Answer from the drawing. Dimensions are ordinates in mm from the lowest x, y and z of the part. A direction names the side the tool comes from. Give positions to 0.01 mm unless a question says otherwise; leave off trailing zeros. Loops run counter-clockwise (first coordinate to the right, second up) from the corner with the lowest first, then second, coordinate; pieces in that order, holes last.
(1) Find section B-B, the plane x = 7.5. Write down the section's boundary in (y, z), then the cut area to 3 significant figures.
(2) Each of these flat-tipped pins is pushed along its axis until it touches: P1, Ø2, axis at x = 8, z = 9, coming from the +Y side; P2, Ø5, axis at x = 7.5, z = 9.5, coming from the +Y side; P3, Ø1, axis at y = 7.5, z = 3, coming from the -X side; P4, Ø1.5, axis at x = 9.5, y = 4, coming from the -Z side. Where does it stop, or does it pass through?
(3) Find section C-C, the plane z = 10. Write down the section's boundary in (x, y).
(4) Which of the six approach directions +Z, -Z, +X, -X, +Y, -Y give full straight-line access (tool end or side, diameter ignored) to the marked faces 1 and 2?
(5) Straight lines are drawn through the part: probe 1 along Z at (x, y) = (10.5, 4); probe 2 along Y at (x, z) = (9.25, 3); probe 3 along X at (y, z) = (2.75, 3.5). For each, find the intervals that lie inside material, in ascending order.
(6) Find section D-D, the plane y = 8.5. Write down the section's boundary in (x, z).
(7) Find section A-A, the plane y = 6.5. Write down the section's boundary in (x, z).
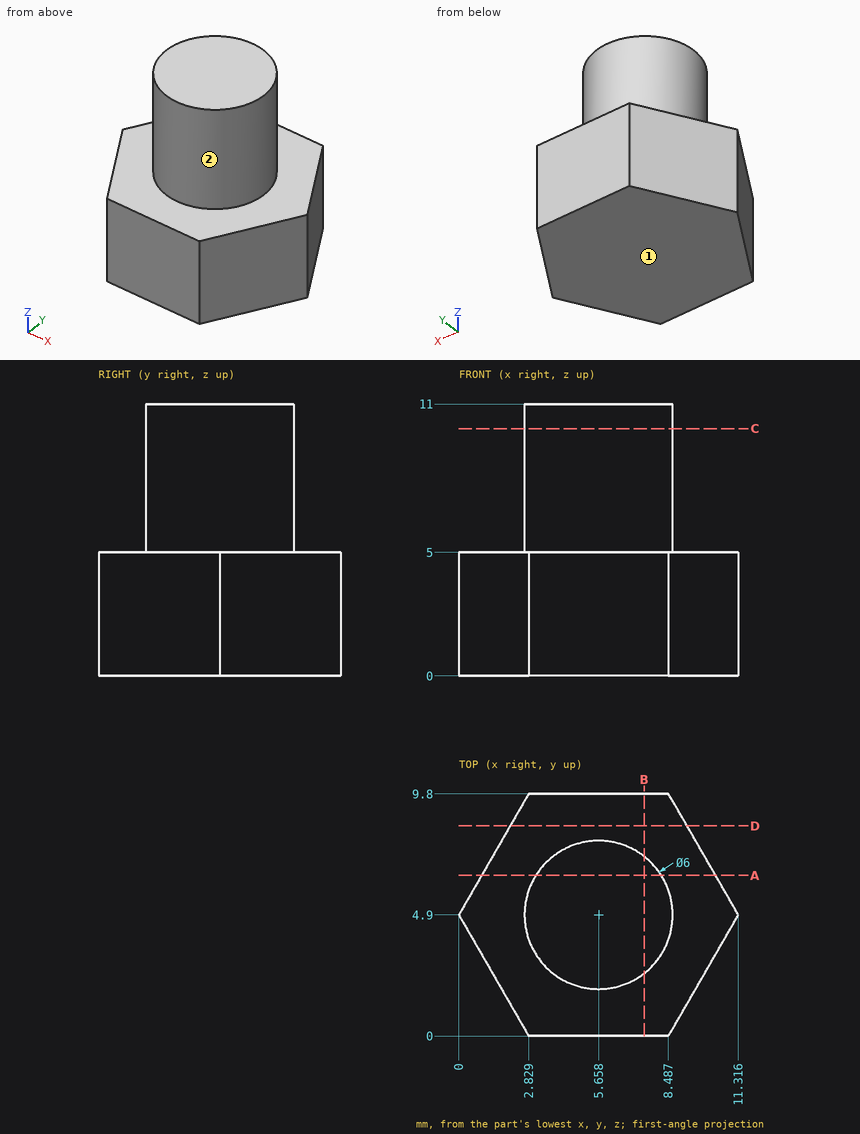
Entries:
1. outline: (0, 0) - (9.8, 0) - (9.8, 5) - (7.27, 5) - (7.27, 11) - (2.53, 11) - (2.53, 5) - (0, 5) - close
1. area: 77.4 mm2
2. P1: stops at y = 7.58
2. P2: stops at y = 7.9
2. P3: stops at x = 1.21
2. P4: stops at z = 0
3. outline: circle Ø6 at (5.66, 4.9)
4. face 1: -Z, +X, -X, +Y, -Y
4. face 2: +Z
5. probe 1: z = 0 to 5
5. probe 2: y = 1.32 to 8.48
5. probe 3: x = 1.24 to 10.07
6. outline: (2.08, 0) - (9.24, 0) - (9.24, 5) - (2.08, 5) - close
7. outline: (0.92, 0) - (10.39, 0) - (10.39, 5) - (8.2, 5) - (8.2, 11) - (3.12, 11) - (3.12, 5) - (0.92, 5) - close
